The listing builds one solid part. Answer for the finished solid, in the listing's coordinates (mm). Coordinates: 2 decimals unless noted, no trailing zeros. Order: outer loops, then holes, each group sorted by start corner. A loop starts at its lowest first (then second) coordinate and runs counter-clockwise, first axis right, second up.
from build123d import *

# Parameters (mm, degrees)
F0_R     = 100
F1_DEPTH = 3
F2_R     = 3
F3_DEPTH = 2
F4_R     = 4.9929816157
F5_DEPTH = 2
F6_R     = 1.99999
F9_DEPTH = 3


# Not quite as in the source:
# - a fillet or chamfer that OpenCascade refuses, or shapes differently, is made with other operations: its cross-section is extruded or revolved along the edge and cut away or added
# - a fillet or chamfer is up to 0.001 mm smaller than in the source, because OpenCascade refuses the exact size


with BuildPart() as f1:
    # F0 (on Top) → F1 (new body)
    with BuildSketch(Plane.XY):
        Circle(F0_R)
    extrude(amount=F1_DEPTH)

    # F2 (on face) → F3 (join)
    with BuildSketch(Plane.XY.offset(3)):
        with Locations((-2.9619428524, 11.0336985157)):
            Circle(F2_R)
        with Locations((9.5783801944, 6.2265754028)):
            Circle(F2_R)
        with Locations((-11.4089615499, 0.5926253015)):
            Circle(F2_R)
        with Locations((-4.0891831618, -10.6674359368)):
            Circle(F2_R)
        with Locations((8.8817073697, -7.1854632832)):
            Circle(F2_R)
    extrude(amount=F3_DEPTH)

    # F4 (on face) → F5 (join)
    with BuildSketch(Plane.XY.offset(3)):
        Circle(F4_R)
    extrude(amount=F5_DEPTH)

    # F6 (radius 2 in the source; OpenCascade refuses exactly that, so slightly less here)
    f6_edges = [f1.edges().sort_by_distance(p)[0] for p in [
        (-5.961943, 11.033699, 5),
        (6.57838, 6.226575, 5),
        (-14.408962, 0.592625, 5),
        (-7.089183, -10.667436, 5),
        (5.881707, -7.185463, 5),
    ]]
    fillet(f6_edges, radius=F6_R)

    # F7: fillet of radius 5 on 1 edges, made by hand

    # F7_s1 → F7_t2 (revolve, cut)
    with BuildSketch(Plane.XZ):
        with BuildLine():
            ThreePointArc((4.9929816157, 3), (3.2290495932, 4.472135955), (0.9929816157, 5))
            Line((0.9929816157, 5), (4.9929816157, 5))
            Line((4.9929816157, 5), (4.9929816157, 3))
        make_face()
    revolve(axis=Axis((0, 0, 5), (0, 0, 1)), mode=Mode.SUBTRACT)

    # F8 (on face) → F9 (cut, through all)
    with BuildSketch(Plane.XY.offset(3)):
        with BuildLine():
            ThreePointArc((66.3999116797, -50.8959301615), (79.2290945271, -26.8718171788), (83.6620820807, 0))
            ThreePointArc((83.6620820807, 0), (82.1834696388, 15.6595432948), (77.7998972031, 30.7655647318))
            Line((77.7998972031, 30.7655647318), (15.2511779268, 2.2686341687))
            Line((15.2511779268, 2.2686341687), (17.7023078517, -2.1256138206))
            Line((17.7023078517, -2.1256138206), (14.2805704694, -5.8146742141))
            Line((14.2805704694, -5.8146742141), (66.3999116797, -50.8959301615))
        make_face()
        with BuildLine():
            Line((9.9430227659, 11.7847964524), (68.923607167, 47.42236132))
            ThreePointArc((68.923607167, 47.42236132), (36.6056794276, 75.2287724991), (-5.2183004193, 83.4991815458))
            Line((-5.2183004193, 83.4991815458), (2.5552738543, 15.2057786606))
            Line((2.5552738543, 15.2057786606), (7.491892841, 16.1790444417))
            Line((7.491892841, 16.1790444417), (9.9430227659, 11.7847964524))
        make_face()
        with BuildLine():
            Line((17.7023078517, -2.1256138206), (15.2511779268, 2.2686341687))
            ThreePointArc((15.2511779268, 2.2686341687), (12.7065485295, -1.5257454222), (14.2805704694, -5.8146742141))
            Line((14.2805704694, -5.8146742141), (17.7023078517, -2.1256138206))
        make_face()
        with BuildLine():
            ThreePointArc((-27.886204899, -78.8777760489), (14.6037462755, -82.3776339354), (53.3012812121, -64.4850168584))
            Line((53.3012812121, -64.4850168584), (6.8704724729, -13.8036856363))
            Line((6.8704724729, -13.8036856363), (3.4487350906, -17.4927460298))
            Line((3.4487350906, -17.4927460298), (-1.1171448371, -15.3784627502))
            Line((-1.1171448371, -15.3784627502), (-27.886204899, -78.8777760489))
        make_face()
        with BuildLine():
            ThreePointArc((2.5552738543, 15.2057786606), (5.3776095614, 11.613164514), (9.9430227659, 11.7847964524))
            Line((9.9430227659, 11.7847964524), (7.491892841, 16.1790444417))
            Line((7.491892841, 16.1790444417), (2.5552738543, 15.2057786606))
        make_face()
        with BuildLine():
            Line((3.4487350906, -17.4927460298), (6.8704724729, -13.8036856363))
            ThreePointArc((6.8704724729, -13.8036856363), (2.4754693095, -12.5561270431), (-1.1171448371, -15.3784627502))
            Line((-1.1171448371, -15.3784627502), (3.4487350906, -17.4927460298))
        make_face()
        with BuildLine():
            Line((-17.7639668564, 54.3390592143), (-23.8027798233, 80.204561284))
            ThreePointArc((-23.8027798233, 80.204561284), (-60.2350372644, 58.0610391212), (-81.0249842257, 20.8397674963))
            Line((-81.0249842257, 20.8397674963), (-55.6504609188, 15.6744066086))
            ThreePointArc((-55.6504609188, 15.6744066086), (-29.7834804383, 28.2223454015), (-17.7639668564, 54.3390592143))
        make_face()
        with BuildLine():
            ThreePointArc((-83.6345341245, 2.1467836063), (-73.8329797706, -39.3450769001), (-44.8578937701, -70.6194969154))
            Line((-44.8578937701, -70.6194969154), (-11.0049924198, -10.799781062))
            Line((-11.0049924198, -10.799781062), (-15.5708723475, -8.6854977824))
            Line((-15.5708723475, -8.6854977824), (-14.971003949, -3.6897384602))
            Line((-14.971003949, -3.6897384602), (-83.6345341245, 2.1467836063))
        make_face()
        with BuildLine():
            Line((-8.1354444491, 13.0980789722), (-17.7639668564, 54.3390592143))
            ThreePointArc((-17.7639668564, 54.3390592143), (-29.7834804383, 28.2223454015), (-55.6504609188, 15.6744066086))
            Line((-55.6504609188, 15.6744066086), (-13.6719318343, 7.1290538689))
            Line((-13.6719318343, 7.1290538689), (-13.0720634358, 12.1248131911))
            Line((-13.0720634358, 12.1248131911), (-8.1354444491, 13.0980789722))
        make_face()
        with BuildLine():
            ThreePointArc((-13.6719318343, 7.1290538689), (-9.3830030423, 8.7030758088), (-8.1354444491, 13.0980789722))
            Line((-8.1354444491, 13.0980789722), (-13.0720634358, 12.1248131911))
            Line((-13.0720634358, 12.1248131911), (-13.6719318343, 7.1290538689))
        make_face()
        with BuildLine():
            Line((-15.5708723475, -8.6854977824), (-11.0049924198, -10.799781062))
            ThreePointArc((-11.0049924198, -10.799781062), (-11.1766243581, -6.2343678575), (-14.971003949, -3.6897384602))
            Line((-14.971003949, -3.6897384602), (-15.5708723475, -8.6854977824))
        make_face()
    extrude(amount=-F9_DEPTH, mode=Mode.SUBTRACT)


solid = f1.part
(1) Given pin 1 Ø10 at (x, y) = (-57.5, -76) entering from +Z; pin 2 Ø3 at (y, z) = (72, 3.5) entering from +X; pin 3 Ø1 at (y, z) = (67.5, 3) entering from +X; pin 4 Ø2 at (x, y) = (73, -63.5) entering from -Z, each flat-ended and moving along its own axis, determine where each tip first touches the part or whether it passes through.
(2) Find the intervals of material crossed by probe 1 along X at (y, z) = (55.5, 2.8); probe 2 along X at (y, z) = (31.5, 0.8); probe 3 along Y at (x, z) = (-58.5, 2.7), in increasing order.
(3) Find section A-A on z = 1.8. Determine the outline of the cut face in (x, y) (1 decimal).
(4) Find section B-B on y = 37.5. Determine the outline of the cut face in (x, z), then the cut area to 3 significant figures.
(5) Find section D-D on x = 46.5. Determine the outline of the cut face in (y, z), then the cut area to 3 significant figures.
(6) The mould has two halves that part along Y. Classify faces 1 (the flat face through (-1, 1, 0)), 2 (the cylindrical face through (95.38, 30.04, 1.48)), 3 (the cylindrical face through (-59.815, 58.494, 1.521)): pulls with the +Y half, pulls with the -Y half, needs draft (parallel to the pull), parting line crosses it, or undercut.
(7) Find section C-C on x = -38.5. Determine the outline of the cut face in (y, z), then the cut area to 3 significant figures.
Resolved:
1. pin 1: stops at z = 3
1. pin 2: stops at x = 70.84
1. pin 3: stops at x = 74.24
1. pin 4: stops at z = 0
2. probe 1: x = -83.19 to -62.6, -18.04 to -2.03, 62.6 to 83.19
2. probe 2: x = -94.91 to -77.51, -12.43 to 0.7, 42.57 to 94.91
2. probe 3: y = -81.1 to -59.81, 0.01 to 16.25, 59.81 to 81.1
3. outline: circle Ø200 at (0, 0); hole (-83.6, 2.1) arc R83.7 ccw to (-44.9, -70.6) - (-11, -10.8) arc R5 ccw to (-15, -3.7) - close; hole (-81, 20.8) - (-13.7, 7.1) arc R5 ccw to (-8.1, 13.1) - (-23.8, 80.2) arc R83.7 ccw to start; hole (-27.9, -78.9) arc R83.7 ccw to (53.3, -64.5) - (6.9, -13.8) arc R5 ccw to (-1.1, -15.4) - close; hole (-5.2, 83.5) - (2.6, 15.2) arc R5 ccw to (9.9, 11.8) - (68.9, 47.4) arc R83.7 ccw to start; hole (14.3, -5.8) - (66.4, -50.9) arc R83.7 ccw to (77.8, 30.8) - (15.3, 2.3) arc R5 ccw to start
4. outline: (-92.7, 0) - (-74.79, 0) - (-74.79, 3) - (-92.7, 3) - close; (-13.83, 0) - (0.02, 0) - (0.02, 3) - (-13.83, 3) - close; (52.5, 0) - (92.7, 0) - (92.7, 3) - (52.5, 3) - close
4. area: 216 mm2
5. outline: (-88.53, 0) - (-69.55, 0) - (-69.55, 3) - (-88.53, 3) - close; (-57.06, 0) - (-33.68, 0) - (-33.68, 3) - (-57.06, 3) - close; (16.51, 0) - (33.87, 0) - (33.87, 3) - (16.51, 3) - close; (69.55, 0) - (88.53, 0) - (88.53, 3) - (69.55, 3) - close
5. area: 236 mm2
6. face 1: needs draft
6. face 2: parting line crosses it
6. face 3: undercut
7. outline: (-92.29, 0) - (-59.38, 0) - (-59.38, 3) - (-92.29, 3) - close; (-1.69, 0) - (12.18, 0) - (12.18, 3) - (-1.69, 3) - close; (74.28, 0) - (92.29, 0) - (92.29, 3) - (74.28, 3) - close
7. area: 194 mm2
